Can you work these out from the model? Positions are in its coordinate system, mm. A direction names the side the tool comes from. Give positions to 0.01 mm unless a question says otherwise; leave off trailing zeros. Loops run counter-clockwise (first coordinate to the right, second up) from the corner with the lowest first, then second, coordinate; pieces in that order, holes last. Notation, with made-up numbers: M 30.5,-38 L 86.5,-38 A15 cw 86.5,-10 Z; hole C 0.5,-39.5 d8. An arc over 180 degrees is marked long. Answer as a JSON object with one key per item and string values.
```python
from build123d import *

# Parameters (mm, degrees)
F3_DEPTH = 621.001
F4_SIZE  = 1
F7_DEPTH = 6


with BuildPart() as f1:
    # F0 (on Front) → F1 (revolve)
    with BuildSketch(Plane.XZ):
        Polygon((12, 79.071932), (0, 79.071932), (0, -663.428068), (15, -663.428068), (15, -625.428068), (13, -625.428068), (13, -623.428068), (15, -623.428068), (15, -593.428068), (17.5, -593.428068), (17.5, -574.428068), (20.5, -574.428068), (20.5, -42.428068), (17.5, -42.428068), (17.5, -23.428068), (15, -23.428068), (15, 1.571932), (13.5, 1.571932), (13.5, 31.571932), (12.5, 31.571932), (12.5, 61.571932), (10, 61.571932), (10, 63.571932), (12, 63.571932), align=None)
    revolve(axis=Axis((0, 0, -292.178068), (0, 0, -1)))

    # F2 (on face) → F3 (cut, through all)
    with BuildSketch(Plane.XY.offset(-42.428068)):
        with BuildLine():
            ThreePointArc((10.677078, 17.5), (0, 20.5), (-10.677078, 17.5))
            Line((-10.677078, 17.5), (0, 17.5))
            Line((0, 17.5), (10.677078, 17.5))
        make_face()
        with BuildLine():
            Line((0, -17.5), (-10.677078, -17.5))
            ThreePointArc((-10.677078, -17.5), (0, -20.5), (10.677078, -17.5))
            Line((10.677078, -17.5), (0, -17.5))
        make_face()
    extrude(amount=-F3_DEPTH, mode=Mode.SUBTRACT)

    # F4
    f4_edges = [f1.edges().sort_by_distance(p)[0] for p in [
        (-15, 0, -663.428068),
        (-17.5, 0, -593.428068),
        (-12, 0, 79.071932),
        (-15, 0, 1.571932),
        (-17.5, 0, -23.428068),
    ]]
    chamfer(f4_edges, length=F4_SIZE)

    # F6 (on offset) → F7 (cut)
    with BuildSketch(Plane.YZ.offset(15)):
        with BuildLine():
            ThreePointArc((4, 51.571932), (0, 55.571932), (-4, 51.571932))
            Line((-4, 51.571932), (-4, 41.571932))
            ThreePointArc((-4, 41.571932), (0, 37.571932), (4, 41.571932))
            Line((4, 41.571932), (4, 51.571932))
        make_face()
    extrude(amount=-F7_DEPTH, mode=Mode.SUBTRACT)


solid = f1.part
```
1) Will these pins go through, and if not, where does the flat tip stop? pin 1 Ø6.5 at (y, z) = (-1.5, 44) entering from +X; pin 2 Ø1.4 at (x, z) = (10.5, 45.5) entering from -Y; pin 3 Ø4 at (x, z) = (-13, -335) entering from -Y.
Answer list:
{"pin 1": "x = 11.84", "pin 2": "y = -7.76", "pin 3": "y = -17.3"}
2) Please list where these lines run through material, in increasing order: line 1 along Z through (x, y) = (11, -7.5); line 2 along Z through (x, y) = (7.5, 8); line 3 along X through (y, z) = (-15.5, -287.5). Write a range as from..to.
Answer list:
{"line 1": "-663.43..-625.43, -623.43..31.57", "line 2": "-663.43..61.57, 63.57..79.07", "line 3": "-13.42..13.42"}
3) Suppose I cut it at B-B, the plane z = -34. Write out the boundary of the cut face in (x, y).
Answer list:
{"outline": "C 0,0 d35"}
4) If we mould it in two halves opening along Z, with no side actions, what happens to faces 1 (the flat face through (0, 17.5, -305)), 2 (the flat face through (0, 0, 79.072)), 3 (the cylindrical face through (-10.316, 7.91, -624.414))? For each: +Z half, -Z half, draft (parallel to the pull), parting line (faces both ways), or undercut.
Answer list:
{"face 1": "draft", "face 2": "+Z half", "face 3": "undercut"}
5) Suppose I cut it at A-A, the plane z = -210. Write out the boundary of the cut face in (x, y).
Answer list:
{"outline": "M -10.68,-17.5 L 10.68,-17.5 A20.5 ccw 10.68,17.5 L -10.68,17.5 A20.5 ccw Z"}
6) For faces 4 (the flat face through (0.1, -13.4, -623.428)), 5 (the cylindrical face through (-14.985, -0.66, -608.218)), 6 (the flat face through (-18, 0, -42.428)), which set-ups out of +Z, -Z, +X, -X, +Y, -Y let a thin tool reach every point of the face, with its end or its side?
Answer list:
{"face 4": "none", "face 5": "-Z", "face 6": "+Z, -X"}
